For this review, take the finished solid that the model builds, in its own axes (mm). A direction names the side the tool comes from. Round coordinates to 2 decimals unless told otherwise and drop trailing zeros. Order: outer loops, then holes, each group sorted by start corner. A loop starts at its lowest first (then second) coordinate and runs counter-clockwise, first axis right, second up. Notation, with made-up numbers: (-22, 74.5) - (17, 74.5) arc R19 cw to (17, 97.5) - close; hole circle Ø7 at (-35, 14). An arc over 180 degrees is marked (long way). One line per item, written item: value.
```python
from build123d import *

# Parameters (mm, degrees)
SKETCH1_R               = 30
BOSS_EXTRUDE1_DEPTH     = 10
SKETCH2_R               = 23.08
BOSS_EXTRUDE2_DEPTH     = 13.486192569
BOSS_EXTRUDE3_DEPTH     = 4
FILLET1_R               = 2
SKETCH5_R               = 1.5
CUT_EXTRUDE1_DEPTH      = 4
MIRROR2_COPY_1_SKETCH_R = 1.5
MIRROR2_COPY_1_DEPTH    = 4
FILLET1_OF_MIRROR2_R    = 2
SKETCH8_R               = 7.5
CUT_EXTRUDE2_DEPTH      = 10


with BuildPart() as part:
    # Sketch1 → Boss-Extrude1 (new body)
    with BuildSketch(Plane.XY):
        Circle(SKETCH1_R)
    extrude(amount=BOSS_EXTRUDE1_DEPTH)

    # Sketch2 → Boss-Extrude2 (add)
    with BuildSketch(Plane.XY.offset(10)):
        Circle(SKETCH2_R)
    extrude(amount=BOSS_EXTRUDE2_DEPTH)

    # Sketch4 → Boss-Extrude3 (add)
    with BuildSketch(Plane(origin=(0, 13, 0), x_dir=(1, 0, 0), z_dir=(0, 1, 0))):
        Polygon((28, -23.486192569), (-28, -23.486192569), (-36.579697763, -30.685413797), (-36.579697763, -35.685413797), (-23.08, -47.013005211), (23.08, -47.013005211), (36.579697763, -35.685413797), (36.579697763, -30.685413797), align=None)
    boss_extrude3 = extrude(amount=-BOSS_EXTRUDE3_DEPTH)

    # Fillet1
    fillet1_edges = [part.edges().sort_by_distance(p)[0] for p in [
        (-36.579697763, 11, 30.685413797),
        (-28, 11, 23.486192569),
        (28, 11, 23.486192569),
        (36.579697763, 11, 30.685413797),
        (36.579697763, 11, 35.685413797),
        (23.08, 11, 47.013005211),
        (-23.08, 11, 47.013005211),
        (-36.579697763, 11, 35.685413797),
    ]]
    fillet(fillet1_edges, radius=FILLET1_R)

    # Sketch5 → Cut-Extrude1 (cut)
    with BuildSketch(Plane(origin=(0, 13, 0), x_dir=(1, 0, 0), z_dir=(0, 1, 0))):
        with Locations(Location((-33.579697763, -33.185413797, 0), (0, 0, 270))):
            Circle(SKETCH5_R)
    cut_extrude1 = extrude(amount=-CUT_EXTRUDE1_DEPTH, mode=Mode.SUBTRACT)

    # Mirror1: Cut-Extrude1 across plane
    add(cut_extrude1.mirror(Plane(origin=(0, 0, 0), x_dir=(0, 0, 1), z_dir=(1, 0, 0))), mode=Mode.SUBTRACT)

    # Mirror2: Boss-Extrude3, Cut-Extrude1 across plane
    add(boss_extrude3.mirror(Plane.ZX))
    add(cut_extrude1.mirror(Plane.ZX), mode=Mode.SUBTRACT)

    # Mirror2 copy 1 sketch → Mirror2 copy 1 (cut)
    with BuildSketch(Plane(origin=(0, -13, 0), x_dir=(-1, 0, 0), z_dir=(0, -1, 0))):
        with Locations(Location((-33.579697763, -33.185413797, 0), (0, 0, 270))):
            Circle(MIRROR2_COPY_1_SKETCH_R)
    extrude(amount=-MIRROR2_COPY_1_DEPTH, mode=Mode.SUBTRACT)

    # Fillet1 of Mirror2
    fillet1_of_mirror2_edges = [part.edges().sort_by_distance(p)[0] for p in [
        (-36.579697763, -11, 30.685413797),
        (-28, -11, 23.486192569),
        (28, -11, 23.486192569),
        (36.579697763, -11, 30.685413797),
        (36.579697763, -11, 35.685413797),
        (23.08, -11, 47.013005211),
        (-23.08, -11, 47.013005211),
        (-36.579697763, -11, 35.685413797),
    ]]
    fillet(fillet1_of_mirror2_edges, radius=FILLET1_OF_MIRROR2_R)

    # Sketch8 → Cut-Extrude2 (cut)
    with BuildSketch(Plane(origin=(0, 0, 0), x_dir=(-1, 0, 0), z_dir=(0, 0, -1))):
        Circle(SKETCH8_R)
    extrude(amount=-CUT_EXTRUDE2_DEPTH, mode=Mode.SUBTRACT)


solid = part.part
```
Item 1: Machinability: for faces 4 (the flat face through (-1, 13, 35)), 5 (the flat face through (-1, -9, 35)), 6 (the flat face through (0, -17, 23.486)), which of the approach directions +Z, -Z, +X, -X, +Y, -Y give a long, thin tool a straight path to every point of the face, cutting with its end or side? Answer none if there is none.
Returned:
face 4: +Z, +X, -X, +Y
face 5: +Z, +X, -X
face 6: +Z, +X, -X, -Y
Item 2: Take a section at D-D (y = 0). Write out the cut boundary in (x, z).
Returned:
outline: (-30, 0) - (-7.5, 0) - (-7.5, 10) - (7.5, 10) - (7.5, 0) - (30, 0) - (30, 10) - (23.08, 10) - (23.08, 23.49) - (-23.08, 23.49) - (-23.08, 10) - (-30, 10) - close
Item 3: Wall thickness on line 1 (Y direction, x = 27, z = 25.5); line 2 (X direction, y = -11, z = 35); line 3 (Y direction, x = 0, z = 6): over which ranges is each line inside the solid? List them lowest first.
Returned:
line 1: -13 to -9, 9 to 13
line 2: -36.56 to 36.56
line 3: -30 to -7.5, 7.5 to 30
Item 4: Take a section at C-C (z = 4). Write out the cut boundary in (x, y).
Returned:
outline: circle Ø60 at (0, 0); hole circle Ø15 at (0, 0)
Item 5: Take a section at A-A (x = -25.5). Write out the cut boundary in (y, z).
Returned:
outline: (-15.8, 0) - (15.8, 0) - (15.8, 10) - (-15.8, 10) - close; (-13, 23.49) - (-9, 23.49) - (-9, 44.98) - (-13, 44.98) - close; (9, 23.49) - (13, 23.49) - (13, 44.98) - (9, 44.98) - close
Item 6: For P1, Ø1.2, axis at x = -22, y = 11.5, coming from the -Z side; P2, Ø5, axis at x = 19, y = 19.5, coming from the +Z side; P3, Ø4, axis at y = -9.5, z = 18.5, coming from the +X side; P4, Ø1.5, axis at x = 4, z = 5, coming from the +Y side, all flat-tipped, find the tip position at first contact; note any pin that passes through.
Returned:
P1: z = 0
P2: z = 10
P3: x = 21.83
P4: y = 29.82
Item 7: The part is to be moulded in two halves that separate along Z. For faces 1 (the flat face through (-32.16, -11.028, 26.977)), 2 (the flat face through (24, 11, 23.486)), 3 (the cylindrical face through (-29.97, 1.32, 4.93)), say which applies: +Z half, -Z half, draft (parallel to the pull), parting line (faces both ways), or undercut.
Returned:
face 1: -Z half
face 2: undercut
face 3: draft
Item 8: Take a section at B-B (x = 0). Write out the cut boundary in (y, z).
Returned:
outline: (-30, 0) - (-7.5, 0) - (-7.5, 10) - (7.5, 10) - (7.5, 0) - (30, 0) - (30, 10) - (23.08, 10) - (23.08, 23.49) - (13, 23.49) - (13, 47.01) - (9, 47.01) - (9, 23.49) - (-9, 23.49) - (-9, 47.01) - (-13, 47.01) - (-13, 23.49) - (-23.08, 23.49) - (-23.08, 10) - (-30, 10) - close
